Can you work these out from the model? Positions are in its coordinate system, mm. Round coordinates to 2 decimals unless told otherwise and drop trailing zeros. Loops run counter-clockwise (first coordinate to the right, second up) from the corner with the lowest first, then second, coordinate; pieces in that order, holes last. Notation, with made-up numbers: (67, 0) - (90, 0) arc R27 ccw to (90, 30) - close; hole circle Ø7 at (5.25, -1). An arc over 180 degrees is marked (long way). Answer as CSV lines item,"result".
```python
from build123d import *

# Parameters (mm, degrees)
SKETCH1_W                            = 127
SKETCH1_H                            = 76.2
BOSS_EXTRUDE1_DEPTH                  = 6.35
CUT_EXTRUDE1_DEPTH                   = 149.24224263
CUT_EXTRUDE1_DEPTH_BACK              = 149.24224263
SKETCH4_R                            = 4.01
F_1_4_0_25_DIAMETER_HOLE1_AT_2_COUNT = 2
F_1_4_0_25_DIAMETER_HOLE1_AT_2_PITCH = 55.88


with BuildPart() as part:
    # Sketch1 → Boss-Extrude1 (new body)
    with BuildSketch(Plane.XY):
        with Locations((-63.5, 38.1)):
            Rectangle(SKETCH1_W, SKETCH1_H)
    extrude(amount=BOSS_EXTRUDE1_DEPTH)

    # Sketch4 → Cut-Extrude1 (cut, two sides: drawn at the far end of the back side and taken through both)
    with BuildSketch(Plane(origin=(0, 0, 0), x_dir=(-1, 0, 0), z_dir=(0, 0, -1)).offset(-CUT_EXTRUDE1_DEPTH_BACK)):
        with Locations((79.912500047, 64.573038165)):
            Circle(SKETCH4_R)
    extrude(amount=CUT_EXTRUDE1_DEPTH + CUT_EXTRUDE1_DEPTH_BACK, mode=Mode.SUBTRACT)

    # Sketch8 → 1/4 (0.25) Diameter Hole1 (revolve, cut)
    with BuildSketch(Plane(origin=(-116.84, 6.35, 0), x_dir=(0, 1, 0), z_dir=(1, 0, 0))):
        Polygon((0, 0), (0, 6.35), (3.175, 6.35), (3.175, 4.105319735), (6.7437, 0), align=None)
    f_1_4_0_25_diameter_hole1 = revolve(axis=Axis((-116.84, 6.35, -6.35), (0, 0, 1)), mode=Mode.SUBTRACT)

    # 1/4 (0.25) Diameter Hole1 at 2: 1/4 (0.25) Diameter Hole1 ×2
    with Locations(*[(i * F_1_4_0_25_DIAMETER_HOLE1_AT_2_PITCH, 0, 0) for i in range(1, F_1_4_0_25_DIAMETER_HOLE1_AT_2_COUNT)]):
        add(f_1_4_0_25_diameter_hole1, mode=Mode.SUBTRACT)


solid = part.part
```
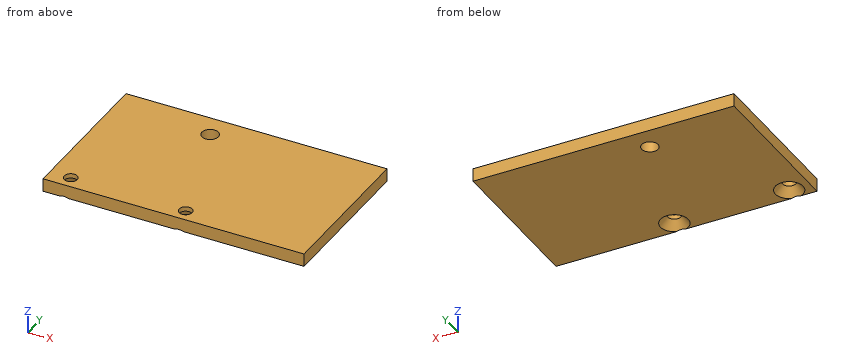
Q1. Imagine slicing it at A-A (y = 6.35). Write out the boundary of the cut face in (x, z) (3 decimals), then the cut area to 3 significant figures.
Checks:
outline,"(-127, 0) - (-123.584, 0) - (-120.015, 4.105) - (-120.015, 6.35) - (-127, 6.35) - close; (-113.665, 4.105) - (-110.096, 0) - (-67.704, 0) - (-64.135, 4.105) - (-64.135, 6.35) - (-113.665, 6.35) - close; (-57.785, 4.105) - (-54.216, 0) - (0, 0) - (0, 6.35) - (-57.785, 6.35) - close"
area,"697 mm²"
Q2. Imagine slicing it at B-B (x = -60.96). Write out the boundary of the cut face in (y, z) (3 decimals).
Checks:
outline,"(0, 0.453) - (3.175, 4.105) - (3.175, 6.35) - (0, 6.35) - close; (9.525, 4.105) - (13.094, 0) - (76.2, 0) - (76.2, 6.35) - (9.525, 6.35) - close"
Q3. If I drill on line 1 along X through (y, z) = (6.35, 4.95) (3 decimals); line 2 along Y through (x, z) = (-60.96, 5.1) (3 decimals); line 3 along X through (y, z) = (5.5, 4.5), over which ranges is the centre line in solid material (lowest first)? Write a range as [from, to].
Checks:
line 1,"[-127, -120.015], [-113.665, -64.135], [-57.785, 0]"
line 2,"[0, 3.175], [9.525, 76.2]"
line 3,"[-127, -119.9], [-113.78, -64.02], [-57.9, 0]"
Q4. Imagine slicing it at C-C (z = 1.75). Write out the boundary of the cut face in (x, y), then the cut area to 3 significant figures.
Checks:
outline,"(-127, 0) - (0, 0) - (0, 76.2) - (-127, 76.2) - close; hole circle Ø10.44 at (-116.84, 6.35); hole circle Ø8.02 at (-79.91, 64.57); hole circle Ø10.44 at (-60.96, 6.35)"
area,"9,460 mm²"
Q5. I'm going to push a flat-ended pin straight in: pin 1 Ø10 at (x, y) = (-116.84, 6.35) entering from -Z. Where does the tip first touch, or does it pass through?
Checks:
pin 1,"z = 2.01"
